Solid Edge part; units mm, degrees
sketch "Sketch1" plane through (0, 0, 0) normal (0, -1, 0) x (1, 0, 0)
  circle A0 centre (2.5, 3.5) radius 1.5
  line L0 (2, 8) -> (5, 4)
  line L1 (5, 0) -> (5, 4)
  line L2 (5, 0) -> (0, 0)
  line L3 (0, 0) -> (0, 8)
  line L4 (0, 8) -> (2, 8)
extrude "Protrusion1" add sketch "Sketch1" against normal blind 5
sketch "Sketch2" plane through (1, 2.5, 8) normal (0, 0, 1) x (1, 0, 0)
  line L0 (-1, 1.5) -> (-1, -1.5)
  line L1 (-1, -1.5) -> (4, -1.5)
  line L2 (4, -1.5) -> (4, 1.5)
  line L3 (4, 1.5) -> (-1, 1.5)
extrude "ExtrudedCutout_1" cut sketch "Sketch2" against normal blind 7 and the other way blind 1
Input: part model. Units: mm. Frame: model coordinates. A direction names the side the tool comes from. Coordinates: 2 decimals unless noted, no trailing zeros. Loops run counter-clockwise (first coordinate to the right, second up) from the corner with the lowest first, then second, coordinate; pieces in that order, holes last. Notation, with made-up numbers: (-11.75, 69.5) - (14.25, 69.5) arc R27 cw to (14.25, 86.5) - close; hole circle Ø11 at (56.25, 18.5). An arc over 180 degrees is marked (long way). Answer in a Markdown table with one row per item. Add a question column.
Item 1: Mould query, pull axis Z, two halves, no side actions, for faces 1 (the flat face through (1, 4.5, 8)), 2 (the flat face through (0.87, 0, 3.06)), 3 (the cylindrical face through (1, 0.49, 3.57)). Classes: released by +Z, released by -Z, zero draft, split by the parting line, or undercut.
Item 2: Section query B-B on y = 4.35. Return the cut outline in (x, z), then the cut area to 3 significant figures.
Item 3: Section query D-D on z = 3.5. Return the cut outline in (x, y), then the cut area to 3 significant figures.
Item 4: Section query A-A on z = 7. Return the cut outline in (x, y), then the cut area to 3 significant figures.
Item 5: Section query C-C on x = 1.2. Return the cut outline in (y, z).
Item 6: Line query: line 1 along Y through (x, z) = (2.7, 6.5); line 2 along Z through (x, y) = (3.1, 0.55); line 3 along Z through (x, y) = (2.5, 4.3). Output: solid intervals per line, ascending. Write a range as [from, to].
Item 7: Access query for faces 4 (the flat face through (1, 1, 5)), 5 (the flat face through (0, 0.8, 3.9)). Directions: +Z, -Z, +X, -X, +Y, -Y. A direction counts if a zero-diameter tool reaches every point of the face in a straight line with its end or side. Return the directions, or none.
Item 8: Contact query for flat-ended pins moving along their axis: P1, Ø2, axis at y = 1.5, z = 5.5, coming from the +X side; P2, Ø2.5, axis at x = 2.5, y = 2, coming from the +Z side. Output: stop coordinate, or through.
Recorded:
| question | item | result |
|---|---|---|
| 1 | face 1 | released by +Z |
| 1 | face 2 | zero draft |
| 1 | face 3 | undercut |
| 2 | outline | (0, 0) - (5, 0) - (5, 4) - (2, 8) - (0, 8) - close; hole circle Ø3 at (2.5, 3.5) |
| 2 | area | 26.9 mm^2 |
| 3 | outline | (0, 0) - (1, 0) - (1, 1) - (0, 1) - close; (0, 4) - (1, 4) - (1, 5) - (0, 5) - close; (4, 0) - (5, 0) - (5, 1) - (4, 1) - close; (4, 4) - (5, 4) - (5, 5) - (4, 5) - close |
| 3 | area | 4.00 mm^2 |
| 4 | outline | (0, 0) - (2.75, 0) - (2.75, 1) - (0, 1) - close; (0, 4) - (2.75, 4) - (2.75, 5) - (0, 5) - close |
| 4 | area | 5.50 mm^2 |
| 5 | outline | (0, 0) - (5, 0) - (5, 2.75) - (4, 2.75) - (4, 1) - (1, 1) - (1, 2.75) - (0, 2.75) - close; (0, 4.25) - (1, 4.25) - (1, 8) - (0, 8) - close; (4, 4.25) - (5, 4.25) - (5, 8) - (4, 8) - close |
| 6 | line 1 | [0, 1], [4, 5] |
| 6 | line 2 | [0, 2.13], [4.87, 6.53] |
| 6 | line 3 | [0, 2], [5, 7.33] |
| 7 | face 4 | +Z, +X, -X |
| 7 | face 5 | +Z, -Z, -X, +Y, -Y |
| 8 | P1 | x = 4.52 |
| 8 | P2 | z = 8 |
